Verification items for the finished model (mm, model axes). A direction names the side the tool comes from. Give positions to 0.01 mm unless a question says otherwise; leave off trailing zeros. Loops run counter-clockwise (first coordinate to the right, second up) from the corner with the lowest first, then second, coordinate; pieces in that order, holes last. Notation, with made-up numbers: (16, 1) - (34, 1) arc R22 ccw to (34, 26) - close; hole circle Ø3 at (62.25, 77). An arc over 180 degrees is marked (long way). One line per item, written item: value. Start each with the question number.
1. Access from +Z, -Z, +X, -X, +Y, -Y to the whole of each face (thin tool, end or side, straight path). Record for faces 1 (the flat face through (0, -14.3, 13.462)), 2 (the cylindrical face through (-0.28, 9.77, 17.52)), 3 (the flat face through (14.3, 0, 13.462)).
2. Scan lines: L1, parallel to X at y = 0, z = 16.95; L2, parallel to X at y = -8.5, z = 17.55; L3, parallel to Y at x = -8.5, z = 17.65. Record each from-to range of solid material in increasing order. Write a range as [from, to].
3. Gauge pin test, flat ends, axial feed: pin 1 (2.5 mm diameter, centred on x = 8.5, y = 0, fed in from -Z); pin 2 (1.5 mm diameter, centred on x = 6, z = 12.5, fed in from -Y); pin 3 (1.1 mm diameter, centred on x = -14, z = 15, fed in from -Y). Record the tip position at first contact, or that the pin passes through.
4. Sectioned sample at A-A (z = 18.25). Count the separate pieces of the cut face and the enclosed holes in it, plus the area to 3 significant figures.
5. Sectioned sample at C-C (z = 6.5). Record the cut outline in (x, y), plus the area to 3 significant figures.
6. Mould release check, pull along Y, two halves, no side actions. Record for faces 4 (the flat face through (3, 14, 15)), 5 (the cylindrical face through (13.856, -5.745, 7.888)), 6 (the flat face through (0, 9, 19)): pulls with the +Y half, pulls with the -Y half, needs draft (parallel to the pull), parting line crosses it, or undercut.
from build123d import *

# Parameters (mm, degrees)
SKETCH_R           = 1.3
POCKET_DEPTH       = 1
SKETCH002_W        = 6
SKETCH002_H        = 2.537703
POCKET001_DEPTH    = 3
POLARPATTERN_COUNT = 4
SKETCH003_R        = 3
SKETCH003_R_2      = 1.3
PAD_DEPTH          = 3
CHAMFER_SIZE       = 0.9


with BuildPart() as part:
    # Sketch001 → Revolution (revolve)
    with BuildSketch(Plane.XZ):
        Polygon((0, 20), (12, 20), (15, 16), (15, 0), (14, 0), (14, 15.999992), (11.749994, 19), (0, 19), align=None)
    revolve(axis=Axis((0, 0, 0), (0, 0, 1)))

    # Sketch (on Face1 of Revolution) → Pocket (cut)
    with BuildSketch(Plane(origin=(0, 0, 20), x_dir=(-1, 0, 0), z_dir=(0, 0, 1))):
        Circle(SKETCH_R)
    extrude(amount=-POCKET_DEPTH, mode=Mode.SUBTRACT)

    # Sketch002 (on DatumPlane) → Pocket001 (cut)
    with BuildSketch(Plane(origin=(0, 15, 8), x_dir=(1, 0, 0), z_dir=(0, 1, 0))):
        with Locations((0, -6.731148)):
            Rectangle(SKETCH002_W, SKETCH002_H)
    pocket001 = extrude(amount=-POCKET001_DEPTH, mode=Mode.SUBTRACT)

    # PolarPattern: Pocket001 ×4 about axis
    polarpattern_axis = Axis((0, 0, 0), (0, 0, 1))
    for i in range(1, POLARPATTERN_COUNT):
        add(pocket001.rotate(polarpattern_axis, i * 360 / POLARPATTERN_COUNT), mode=Mode.SUBTRACT)

    # Sketch003 (on Face9 of PolarPattern) → Pad (join)
    with BuildSketch(Plane(origin=(0, 0, 19), x_dir=(1, 0, 0), z_dir=(0, 0, -1))):
        with Locations((-8.5, 0)):
            Circle(SKETCH003_R)
        with Locations((-8.5, 0)):
            Circle(SKETCH003_R_2, mode=Mode.SUBTRACT)
        with Locations((0, 8.5)):
            Circle(SKETCH003_R)
        with Locations((0, 8.5)):
            Circle(SKETCH003_R_2, mode=Mode.SUBTRACT)
        with Locations((8.5, 0)):
            Circle(SKETCH003_R)
        with Locations((8.5, 0)):
            Circle(SKETCH003_R_2, mode=Mode.SUBTRACT)
        with Locations((0, -8.5)):
            Circle(SKETCH003_R)
        with Locations((0, -8.5)):
            Circle(SKETCH003_R_2, mode=Mode.SUBTRACT)
    extrude(amount=PAD_DEPTH)

    # Chamfer
    chamfer_edges = [part.edges().sort_by_distance(p)[0] for p in [
        (1.3, 0, 20),
    ]]
    chamfer(chamfer_edges, length=CHAMFER_SIZE)


solid = part.part
Results are:
1. face 1: +Y, -Y
1. face 2: -Z
1. face 3: +X, -X
2. L1: x = [-14.29, -13.29], [-11.5, -9.8], [-7.2, -5.5], [5.5, 7.2], [9.8, 11.5], [13.29, 14.29]
2. L2: x = [-10.92, -9.62], [-3, -1.3], [1.3, 3], [9.62, 10.92]
2. L3: y = [-10.82, -9.52], [-3, -1.3], [1.3, 3], [9.52, 10.82]
3. pin 1: stops at z = 19
3. pin 2: stops at y = -14.05
3. pin 3: stops at y = -6.64
4. separate pieces: 5
4. enclosed holes: 5
4. area: 172 mm^2
5. outline: circle Ø30 at (0, 0); hole circle Ø28 at (0, 0)
5. area: 91.1 mm^2
6. face 4: needs draft
6. face 5: parting line crosses it
6. face 6: undercut
